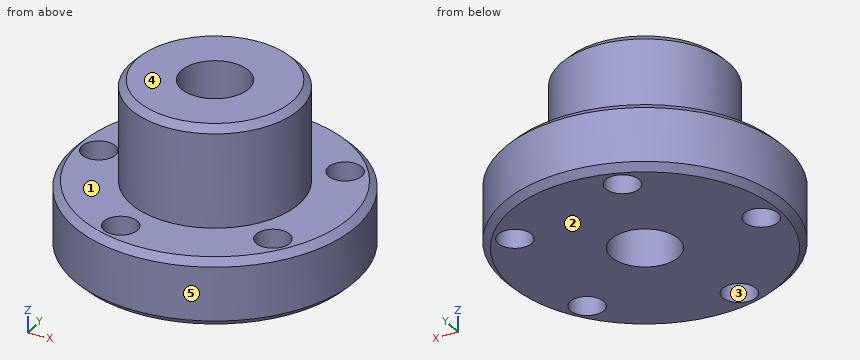
```python
from build123d import *

# Parameters (mm, degrees)
F3_D     = 5
F3_DEPTH = 20


with BuildPart() as f1:
    # F0 (on Front) → F1 (revolve)
    with BuildSketch(Plane.XZ):
        Polygon((-5, 0), (-5, 25), (-11.5, 25), (-12.5, 24), (-12.5, 16), (-12.5, 10), (-20, 10), (-21, 9), (-21, 1), (-20, 0), align=None)
    revolve(axis=Axis((0, 0, 12.5), (0, 0, 1)))

    # F3
    with Locations(Plane.XY.offset(10)):
        with Locations((-17, 0), (-5.253289, 16.167961), (13.753289, 9.992349), (13.753289, -9.992349), (-5.253289, -16.167961)):
            Hole(F3_D / 2, depth=F3_DEPTH)


solid = f1.part
```
Geometry: final body of the model. Coordinates: model frame, mm. Face numbers are marked on the shaded views. A direction names the side the tool comes from. Coordinates: 2 decimals unless noted, no trailing zeros. Order: outer loops, then holes, each group sorted by start corner. A loop starts at its lowest first (then second) coordinate and runs counter-clockwise, first axis right, second up. Notation, with made-up numbers: (84, -30.75) -> (141, -30.75) arc R20 ccw to (141, -19.75) -> close; hole circle Ø4 at (69, -13). An arc over 180 degrees is marked (long way). Answer in a Markdown table with one row per item.
Item 1: Section A-A on y = 0. Output: boundary loops of the cut face in (x, z), plus the area to 3 significant figures.
Return value:
| item | result |
|---|---|
| outline | (-21, 1) -> (-20, 0) -> (-19.5, 0) -> (-19.5, 10) -> (-20, 10) -> (-21, 9) -> close; (-14.5, 0) -> (-5, 0) -> (-5, 25) -> (-11.5, 25) -> (-12.5, 24) -> (-12.5, 10) -> (-14.5, 10) -> close; (5, 0) -> (20, 0) -> (21, 1) -> (21, 9) -> (20, 10) -> (12.5, 10) -> (12.5, 24) -> (11.5, 25) -> (5, 25) -> close |
| area | 492 mm² |
Item 2: Draft query along Y for the marked faces 3, 4 and 5. Return one class per face: released by +Y, released by -Y, zero draft, split by the parting line, or undercut.
Return value:
| item | result |
|---|---|
| face 3 | undercut |
| face 4 | zero draft |
| face 5 | split by the parting line |
Item 3: Access query for the marked faces 1 and 2. Directions: +Z, -Z, +X, -X, +Y, -Y. A direction counts if a zero-diameter tool reaches every point of the face in a straight line with its end or side. Return the directions, or none.
Return value:
| item | result |
|---|---|
| face 1 | +Z |
| face 2 | -Z, +X, -X, +Y, -Y |
Item 4: Ray query, L1, parallel to Y at x = 0, z = 19.75; L2, parallel to Z at x = -18, y = -8; L3, parallel to X at y = 0.5, z = 3.25. Return the intervals inside material, ascending.
Return value:
| item | result |
|---|---|
| L1 | y = -12.5 to -5, 5 to 12.5 |
| L2 | z = 0 to 10 |
| L3 | x = -20.99 to -19.45, -14.55 to -4.97, 4.97 to 20.99 |
Item 5: Contact query for flat-ended pins moving along their axis: P1, Ø12, axis at y = -10, z = 11, coming from the -X side; P2, Ø4, axis at x = -7.5, z = 14, coming from the -Y side (3 decimals); P3, Ø10, axis at x = -11.5, y = -15.5, coming from the +Z side. Output: stop coordinate, or through.
Return value:
| item | result |
|---|---|
| P1 | stops at x = -20.55 |
| P2 | stops at y = -11.225 |
| P3 | stops at z = 10 |
Item 6: Section C-C on z = 16. Output: boundary loops of the cut face in (x, y).
Return value:
| item | result |
|---|---|
| outline | circle Ø25 at (0, 0); hole circle Ø10 at (0, 0) |
Item 7: Section B-B on x = 0. Output: boundary loops of the cut face in (y, z), plus the area to 3 significant figures.
Return value:
| item | result |
|---|---|
| outline | (-21, 1) -> (-20, 0) -> (-5, 0) -> (-5, 25) -> (-11.5, 25) -> (-12.5, 24) -> (-12.5, 10) -> (-20, 10) -> (-21, 9) -> close; (5, 0) -> (20, 0) -> (21, 1) -> (21, 9) -> (20, 10) -> (12.5, 10) -> (12.5, 24) -> (11.5, 25) -> (5, 25) -> close |
| area | 542 mm² |
